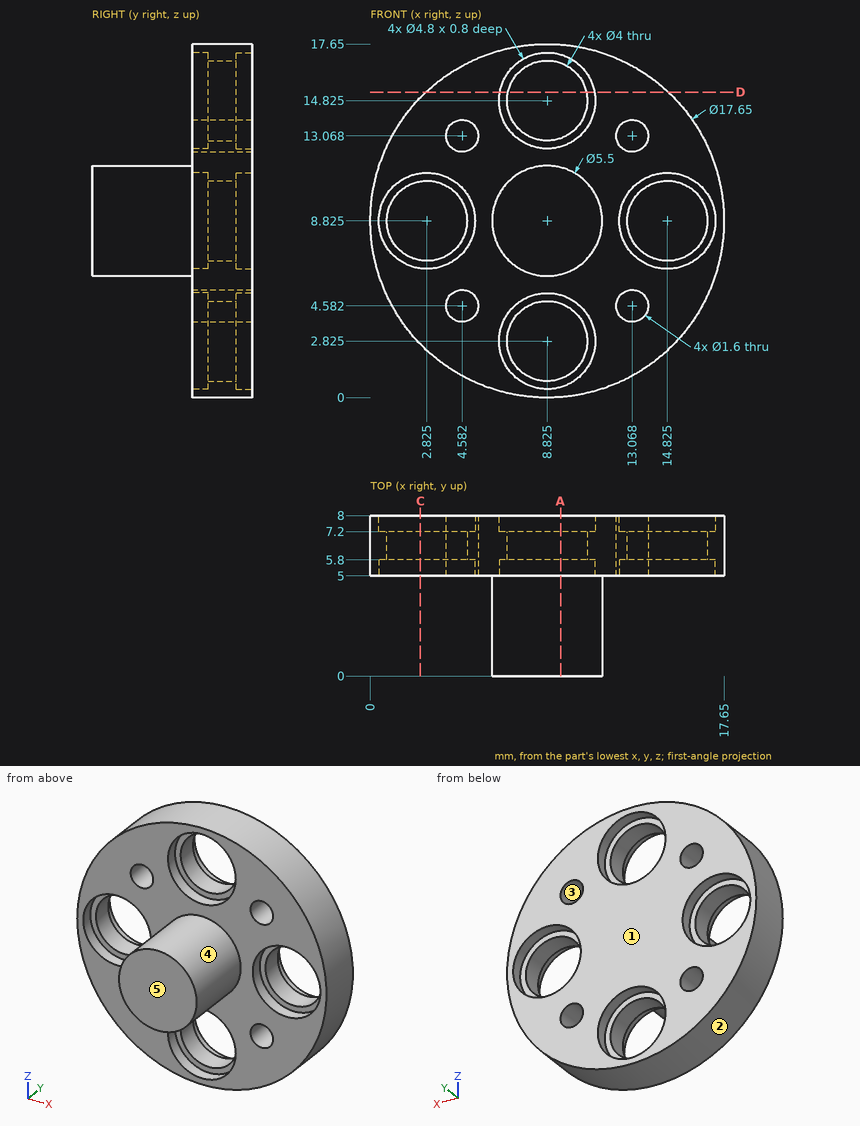
Input: dimensioned drawing with shaded views. Units: mm. Origin: part minimum x, y, z. A direction names the side the tool comes from. Give positions to 0.01 mm unless a question says otherwise; leave off trailing zeros. Write each loop counter-clockwise with the first axis right and the second up, starting at its lowest first coordinate (ties: lowest second). Pieces come first, ordered by that corner, then holes.
Q1. Pull-direction query (Z, two-part tool) for the marked faces 1, 2 and 3; classes: pulls with the +Z half, pulls with the -Z half, needs draft (parallel to the pull), parting line crosses it, or undercut.
Q2. Section D-D, the plane z = 15.25. Output: boundary loops of the cut face in (x, y) (1 decimal).
Q3. Section C-C, the plane x = 2.5. Output: boundary loops of the cut face in (y, z).
Q4. Material intervals for probe 1 along Y at (x, z) = (15.75, 11.25); probe 2 along Y at (x, z) = (2.5, 11); probe 3 along X at (y, z) = (6.75, 14.75) (1 decimal), sorted ascending.
Q5. First-contact query: P1, Ø1, axis at x = 4.58, z = 13.07, coming from the +Y side; P2, Ø2, axis at x = 13.07, z = 4.58, coming from the +Y side; P3, Ø4, axis at y = 5.5, z = 5.5, coming from the +X side; P4, Ø4, axis at x = 8.5, z = 15, coming from the -Y side. Flat tips, straight axial feed; report the tip coordinate or a pass-through.
Q6. Set-up query: the marked faces 4 and 5. Return all of +Z, -Z, +X, -X, +Y, -Y with unobstructed straight access to the full face (end or side cutting, diameter ignored); none if empty.
Q7. Section A-A, the plane x = 9.5. State how many separate pieces and enclosed holes the cut face has.
Filled in:
1. face 1: needs draft
1. face 2: parting line crosses it
1. face 3: undercut
2. outline: (2.8, 5) - (6.5, 5) - (6.5, 5.8) - (6.9, 5.8) - (6.9, 7.2) - (6.5, 7.2) - (6.5, 8) - (2.8, 8) - close; (10.8, 5.8) - (11.2, 5.8) - (11.2, 5) - (14.9, 5) - (14.9, 8) - (11.2, 8) - (11.2, 7.2) - (10.8, 7.2) - close
3. outline: (5, 2.67) - (8, 2.67) - (8, 6.45) - (7.2, 6.45) - (7.2, 6.85) - (5.8, 6.85) - (5.8, 6.45) - (5, 6.45) - close; (5, 11.2) - (5.8, 11.2) - (5.8, 10.8) - (7.2, 10.8) - (7.2, 11.2) - (8, 11.2) - (8, 14.98) - (5, 14.98) - close
4. probe 1: y = 5 to 8
4. probe 2: y = 5.8 to 7.2
4. probe 3: x = 2.3 to 6.8, 10.8 to 15.4
5. P1: passes through
5. P2: stops at y = 8
5. P3: stops at x = 17.55
5. P4: stops at y = 5.8
6. face 4: -Y
6. face 5: +Z, -Z, +X, -X, -Y
7. separate pieces: 3
7. enclosed holes: 0
